Design review of the part shown in the three views and the two pictorial views. Dimensions are in mm from the part's minimum x, y and z. Give positions to 0.01 mm unless a question says otherwise; leave off trailing zeros. Loops run counter-clockwise (first coordinate to the right, second up) from the corner with the lowest first, then second, coordinate; pieces in that order, holes last. Notation, with made-up numbers: (20, 35.5) -> (32, 35.5) arc R35 ccw to (32, 71.5) -> close; hole circle Ø2 at (55, 41). An arc over 180 degrees is marked (long way). Answer as CSV lines item,"result". Start each with the question number.
Item 1: Add section C-C on z = 48. State the section outline as (x, y) points, plus the area to 3 significant figures.
Item 2: Add section D-D on y = 0.85. State the section outline as (x, z) points (3 decimals), plus the area to 3 significant figures.
Item 3: For L1, parallel to Z at x = 34.5, y = 0.2; L2, parallel to Z at x = 3.5, y = 1.25 (3 decimals); L3, parallel to X at y = 0.45, z = 44, list the stretches that pass through material, from the lowest coordinate up. Write a range as from..to.
Item 4: Clearance check with a flat-ended pin moving along its axis: P1, Ø0.6, axis at x = 23.5, y = 1.5, coming from the -Z side. State where the tip first meets the part, or that it passes through.
Item 5: Add section B-B on z = 24.5. State the section outline as (x, y) points.
Item 6: Add section A-A on x = 42.5. State the section outline as (y, z) points.
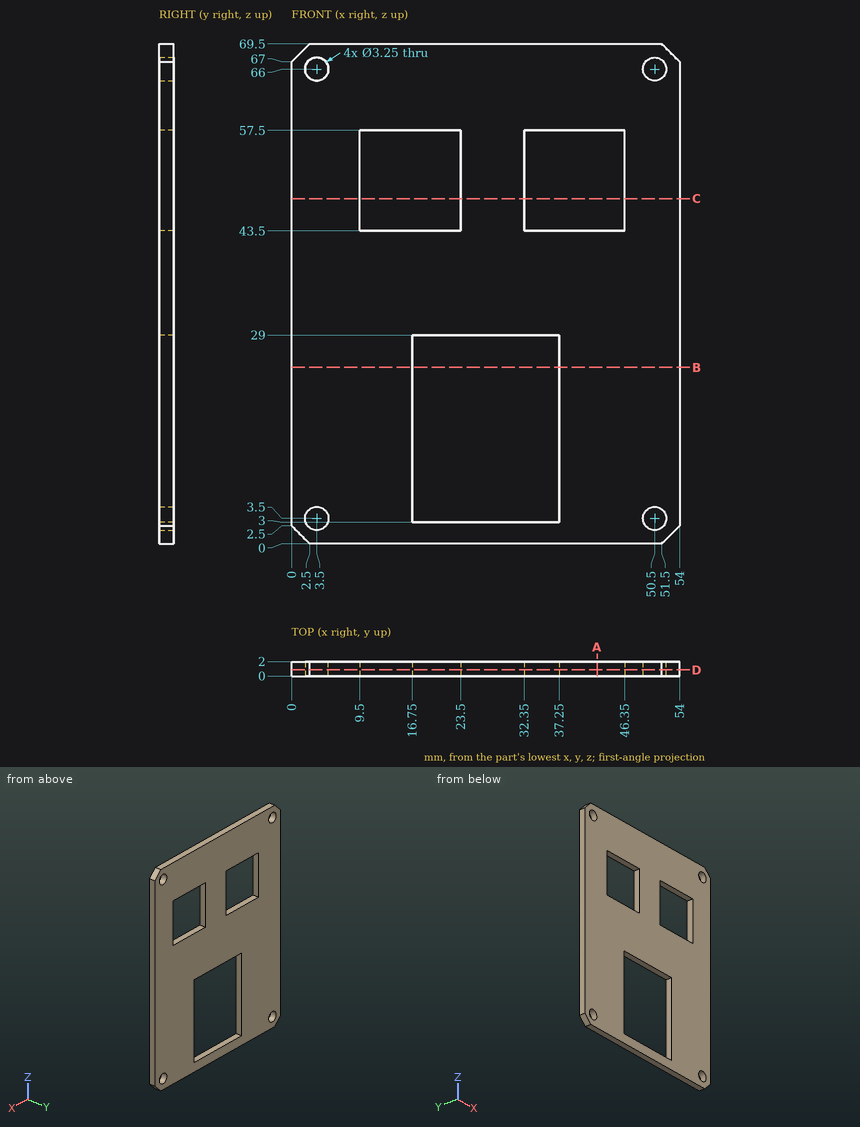
Computed values:
1,outline,"(0, 0) -> (9.5, 0) -> (9.5, 2) -> (0, 2) -> close; (23.5, 0) -> (32.35, 0) -> (32.35, 2) -> (23.5, 2) -> close; (46.35, 0) -> (54, 0) -> (54, 2) -> (46.35, 2) -> close"
1,area,"52.0 mm²"
2,outline,"(0, 2.5) -> (2.5, 0) -> (51.5, 0) -> (54, 2.5) -> (54, 67) -> (51.5, 69.5) -> (2.5, 69.5) -> (0, 67) -> close; hole circle Ø3.25 at (3.5, 3.5); hole circle Ø3.25 at (3.5, 66); hole (9.5, 43.5) -> (23.5, 43.5) -> (23.5, 57.5) -> (9.5, 57.5) -> close; hole (16.75, 3) -> (37.25, 3) -> (37.25, 29) -> (16.75, 29) -> close; hole (32.35, 43.5) -> (46.35, 43.5) -> (46.35, 57.5) -> (32.35, 57.5) -> close; hole circle Ø3.25 at (50.5, 3.5); hole circle Ø3.25 at (50.5, 66)"
2,area,"2,780 mm²"
3,L1,"0..3, 29..43.5, 57.5..69.5"
3,L2,"0..1.875, 5.125..64.375, 67.625..69.5"
3,L3,"0..9.5, 23.5..32.35, 46.35..54"
4,P1,"z = 0"
5,outline,"(0, 0) -> (16.75, 0) -> (16.75, 2) -> (0, 2) -> close; (37.25, 0) -> (54, 0) -> (54, 2) -> (37.25, 2) -> close"
6,outline,"(0, 0) -> (2, 0) -> (2, 43.5) -> (0, 43.5) -> close; (0, 57.5) -> (2, 57.5) -> (2, 69.5) -> (0, 69.5) -> close"
